Source: CAD feature listing. Evaluate the final solid. Frame: model axes, mm. A direction names the side the tool comes from. Coordinates: 2 decimals unless noted, no trailing zeros. Order: outer loops, then holes, each group sorted by start corner. A loop starts at its lowest first (then second) coordinate and runs counter-clockwise, first axis right, second up. Notation, with made-up numbers: (87, 57.25) - (143, 57.25) arc R20 cw to (143, 65.25) - close; hole circle Ø4 at (60, -33.5). An arc over 180 degrees is marked (long way). One line per question, with ' | ' between items.
from build123d import *

# Parameters (mm, degrees)
SKETCH2_W           = 31.77
SKETCH2_H           = 15.78
BOSS_EXTRUDE2_DEPTH = 9.65
SKETCH3_R           = 2.45
BOSS_EXTRUDE3_DEPTH = 1.76
SHELL1_T            = -1.2
SKETCH4_R           = 3.215
SKETCH4_R_2         = 2.305
BOSS_EXTRUDE4_DEPTH = 8.25


with BuildPart() as part:
    # Sketch2 → Boss-Extrude2 (new body)
    with BuildSketch(Plane(origin=(0, 0, 0), x_dir=(1, 0, 0), z_dir=(0, 1, 0))):
        Rectangle(SKETCH2_W, SKETCH2_H)
    extrude(amount=-BOSS_EXTRUDE2_DEPTH)

    # Sketch3 → Boss-Extrude3 (add)
    with BuildSketch(Plane(origin=(0, 0, 0), x_dir=(1, 0, 0), z_dir=(0, 1, 0))):
        with Locations(Location((-11.9125, 3.945, 0), (0, 0, 270))):
            Circle(SKETCH3_R)
        with Locations(Location((-3.9675, 3.945, 0), (0, 0, 270))):
            Circle(SKETCH3_R)
        with Locations(Location((-3.9675, -3.945, 0), (0, 0, 270))):
            Circle(SKETCH3_R)
        with Locations(Location((-11.9125, -3.945, 0), (0, 0, 270))):
            Circle(SKETCH3_R)
        with Locations(Location((11.9125, -3.945, 0), (0, 0, 90))):
            Circle(SKETCH3_R)
        with Locations(Location((3.9675, -3.945, 0), (0, 0, 90))):
            Circle(SKETCH3_R)
        with Locations(Location((3.9675, 3.945, 0), (0, 0, 90))):
            Circle(SKETCH3_R)
        with Locations(Location((11.9125, 3.945, 0), (0, 0, 90))):
            Circle(SKETCH3_R)
    extrude(amount=BOSS_EXTRUDE3_DEPTH)

    # Shell1
    shell1_openings = [part.faces().sort_by_distance(p)[0] for p in [
        (0, -9.65, 0),
    ]]
    offset(amount=SHELL1_T, openings=shell1_openings, kind=Kind.INTERSECTION)

    # Sketch4 → Boss-Extrude4 (add)
    # profile 1 of 3: a face of its own
    with BuildSketch(Plane.XZ.offset(1.2)):
        with Locations(Location((0, 0, 0), (0, 0, 90))):
            Circle(SKETCH4_R)
        with Locations(Location((0, 0, 0), (0, 0, 90))):
            Circle(SKETCH4_R_2, mode=Mode.SUBTRACT)
    # profile 2 of 3: a face of its own
    with BuildSketch(Plane.XZ.offset(1.2)):
        with Locations(Location((7.945, 0, 0), (0, 0, 90))):
            Circle(SKETCH4_R)
        with Locations(Location((7.945, 0, 0), (0, 0, 90))):
            Circle(SKETCH4_R_2, mode=Mode.SUBTRACT)
    # profile 3 of 3: a face of its own
    with BuildSketch(Plane.XZ.offset(1.2)):
        with Locations(Location((-7.945, 0, 0), (0, 0, 90))):
            Circle(SKETCH4_R)
        with Locations(Location((-7.945, 0, 0), (0, 0, 90))):
            Circle(SKETCH4_R_2, mode=Mode.SUBTRACT)
    extrude(amount=BOSS_EXTRUDE4_DEPTH)


solid = part.part
(1) Pin query (flat end, axial travel): P1, Ø3, axis at x = -9, z = 0.5, coming from the -Y side; P2, Ø3, axis at x = -11.5, z = -4, coming from the -Y side; P3, Ø6, axis at x = 7.945, z = 0, coming from the +Y side. Return the tip coordinate at first contact, or that it passes through.
Taken from the geometry:
P1: stops at y = -9.45 | P2: stops at y = -1.2 | P3: stops at y = 0
(2) Set-up query: faces 4 (the cylindrical face through (-13.13, -0.33, 3.67)), 5 (the cylindrical face through (3.23, 0.87, -6.28)), 6 (the flat face through (15.885, -5, 0)). Return all of +Z, -Z, +X, -X, +Y, -Y with unobstructed straight access to the full face (end or side cutting, diameter ignored); none if empty.
Taken from the geometry:
face 4: -Y | face 5: +Y | face 6: +Z, -Z, +X, +Y, -Y
(3) Cut plane A-A (y = -7.25). Return the cut outline in (x, z) (3 decimals).
Taken from the geometry:
outline: (-15.885, -7.89) - (15.885, -7.89) - (15.885, 7.89) - (-15.885, 7.89) - close; circle Ø6.43 at (-7.945, 0); circle Ø6.43 at (0, 0); circle Ø6.43 at (7.945, 0); hole (-14.685, -6.69) - (14.685, -6.69) - (14.685, 6.69) - (-14.685, 6.69) - close; hole circle Ø4.61 at (-7.945, 0); hole circle Ø4.61 at (0, 0); hole circle Ø4.61 at (7.945, 0)
(4) Material intervals for L1, parallel to Z at x = 12, y = -0.75; L2, parallel to Z at x = 13.5, y = -7.75; L3, parallel to X at y = 1.25, z = -1.75, sorted ascending. Write a range as from..to.
Taken from the geometry:
L1: z = -7.89..-5.19, -2.7..2.7, 5.19..7.89 | L2: z = -7.89..-6.69, 6.69..7.89 | L3: x = -13..-10.82, -5.06..-2.88, 2.88..5.06, 10.82..13
(5) Cut plane D-D (z = 5.75). Return the cut outline in (x, y) (3 decimals).
Taken from the geometry:
outline: (-15.885, -9.65) - (-14.685, -9.65) - (-14.685, -1.2) - (14.685, -1.2) - (14.685, -9.65) - (15.885, -9.65) - (15.885, 0) - (13.569, 0) - (13.569, 1.76) - (10.256, 1.76) - (10.256, 0) - (5.624, 0) - (5.624, 1.76) - (2.311, 1.76) - (2.311, 0) - (-2.311, 0) - (-2.311, 1.76) - (-5.624, 1.76) - (-5.624, 0) - (-10.256, 0) - (-10.256, 1.76) - (-13.569, 1.76) - (-13.569, 0) - (-15.885, 0) - close
(6) Cut plane C-C (x = 0). Return the cut outline in (y, z) (3 decimals), and give its area (3 significant figures).
Taken from the geometry:
outline: (-9.65, -7.89) - (0, -7.89) - (0, 7.89) - (-9.65, 7.89) - (-9.65, 6.69) - (-1.2, 6.69) - (-1.2, 3.215) - (-9.45, 3.215) - (-9.45, 2.305) - (-1.2, 2.305) - (-1.2, -2.305) - (-9.45, -2.305) - (-9.45, -3.215) - (-1.2, -3.215) - (-1.2, -6.69) - (-9.65, -6.69) - close | area: 54.2 mm²
(7) Pull-direction query (Z, two-part tool) for faces 1 (the flat face through (0, -5, 7.89)), 2 (the flat face through (-12, 1.76, -4)), 3 (the cylindrical face through (1.96, -5.27, -2.55)); classes: pulls with the +Z half, pulls with the -Z half, needs draft (parallel to the pull), parting line crosses it, or undercut.
Taken from the geometry:
face 1: pulls with the +Z half | face 2: needs draft | face 3: undercut
